from build123d import *

# Parameters (mm, degrees)
CROQUIS1_R              = 53.34
CROQUIS1_R_2            = 50.8254
SALIENTE_EXTRUIR1_DEPTH = 9.525
CROQUIS2_R              = 7.45617
SALIENTE_EXTRUIR2_DEPTH = 99.06
CROQUIS3_R              = 50.8254
CORTAR_EXTRUIR1_DEPTH   = 49.53


with BuildPart() as part:
    # Croquis1 → Saliente-Extruir1 (new, symmetric)
    with BuildSketch(Plane(origin=(0, 0, 0), x_dir=(1, 0, 0), z_dir=(0, 1, 0))):
        with Locations(Location((0, 0, 0), (0, 0, 90))):
            Circle(CROQUIS1_R)
        with Locations(Location((0, 0, 0), (0, 0, 90))):
            Circle(CROQUIS1_R_2, mode=Mode.SUBTRACT)
    extrude(amount=SALIENTE_EXTRUIR1_DEPTH, both=True)

    # Croquis2 → Saliente-Extruir2 (add)
    with BuildSketch(Plane(origin=(0, 0, 0), x_dir=(0, 0, -1), z_dir=(1, 0, 0))):
        with Locations(Location((0, 0, 0), (0, 0, 180))):
            Circle(CROQUIS2_R)
    extrude(amount=SALIENTE_EXTRUIR2_DEPTH)

    # Croquis3 → Cortar-Extruir1 (cut, symmetric)
    with BuildSketch(Plane.XZ.offset(9.525)):
        with Locations(Location((0, 0, 0), (0, 0, 270))):
            Circle(CROQUIS3_R)
    extrude(amount=CORTAR_EXTRUIR1_DEPTH, both=True, mode=Mode.SUBTRACT)


solid = part.part
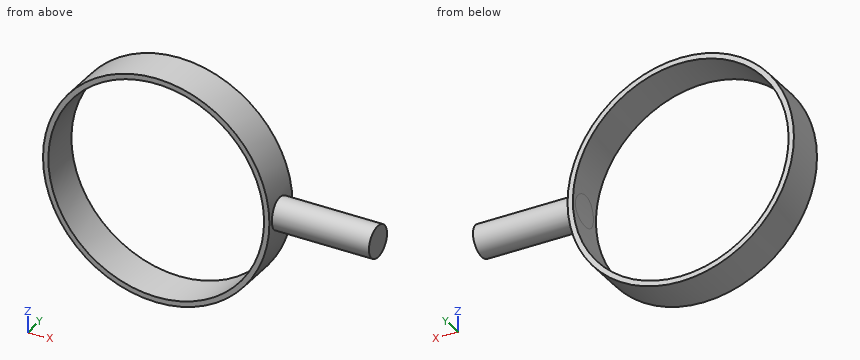
Here's how the part is built. I have some questions about the finished solid (model axes, mm). Round coordinates to 2 decimals unless told otherwise and drop trailing zeros. Order: outer loops, then holes, each group sorted by start corner. A loop starts at its lowest first (then second) coordinate and runs counter-clockwise, first axis right, second up. Notation, with made-up numbers: M 29.5,40 L 86.5,40 A23 cw 86.5,65 Z; hole C -7.5,-10 d8. An arc over 180 degrees is marked long. One line per question, with ' | ' between items.
1) I'm going to push flat-ended pins straight in: pin 1 Ø3 at (y, z) = (-6.5, -19.5) entering from +X; pin 2 Ø6 at (y, z) = (4.5, 33) entering from -X; pin 3 Ø8 at (x, y) = (-25.5, 1.5) entering from -Z (3 decimals). Where does each tip first touch, or does it pass through?
Checked values:
pin 1: stops at x = 50.21 | pin 2: stops at x = -44.1 | pin 3: stops at z = -48.815
2) Imagine slicing it at A-A, the plane z = 0. Write out the boundary of the cut face in (x, y) (3 decimals), plus the area to 3 significant figures.
Checked values:
outline: M -53.34,-9.525 L -50.825,-9.525 L -50.825,9.525 L -53.34,9.525 Z; M 50.825,-9.525 L 53.34,-9.525 L 53.34,-7.456 L 99.06,-7.456 L 99.06,7.456 L 53.34,7.456 L 53.34,9.525 L 50.825,9.525 Z | area: 778 mm²
3) I need wall thicknesses on line 1 (X direction, y = -2, z = 0); line 2 (X direction, y = 2.75, z = -42); line 3 (Z direction, x = 1.5, y = 1). Which ranges of each line are inside material? Lowest first, please.
Checked values:
line 1: x = -53.34 to -50.83, 50.83 to 99.06 | line 2: x = -32.88 to -28.62, 28.62 to 32.88 | line 3: z = -53.32 to -50.8, 50.8 to 53.32
4) Imagine slicing it at D-D, the plane x = 60. Write out the boundary of the cut face in (y, z), plus the area to 3 significant figures.
Checked values:
outline: C 0,0 d14.91 | area: 175 mm²
5) Imagine slicing it at C-C, the plane y = 0. Write out the boundary of the cut face in (x, z).
Checked values:
outline: M 52.82,-7.46 L 99.06,-7.46 L 99.06,7.46 L 52.82,7.46 A53.34 ccw long Z; hole C 0,0 d101.65
6) Imagine slicing it at B-B, the plane x = 0. Write out the boundary of the cut face in (y, z) (3 decimals), plus the area to 3 significant figures.
Checked values:
outline: M -9.525,-53.34 L 9.525,-53.34 L 9.525,-50.825 L -9.525,-50.825 Z; M -9.525,50.825 L 9.525,50.825 L 9.525,53.34 L -9.525,53.34 Z | area: 95.8 mm²
